Design review of the part shown in the three views and the two pictorial views. Dimensions are in mm from the part's minimum x, y and z. Coordinates: 2 decimals unless noted, no trailing zeros. Loops run counter-clockwise (first coordinate to the right, second up) from the corner with the lowest first, then second, coordinate; pieces in that order, holes last. Notation, with made-up numbers: (43, 51) -> (51, 51) arc R24 cw to (51, 72) -> close; hole circle Ø9 at (-37.75, -14). An arc over 180 degrees is marked (long way). Answer in a Markdown table with one row per item.
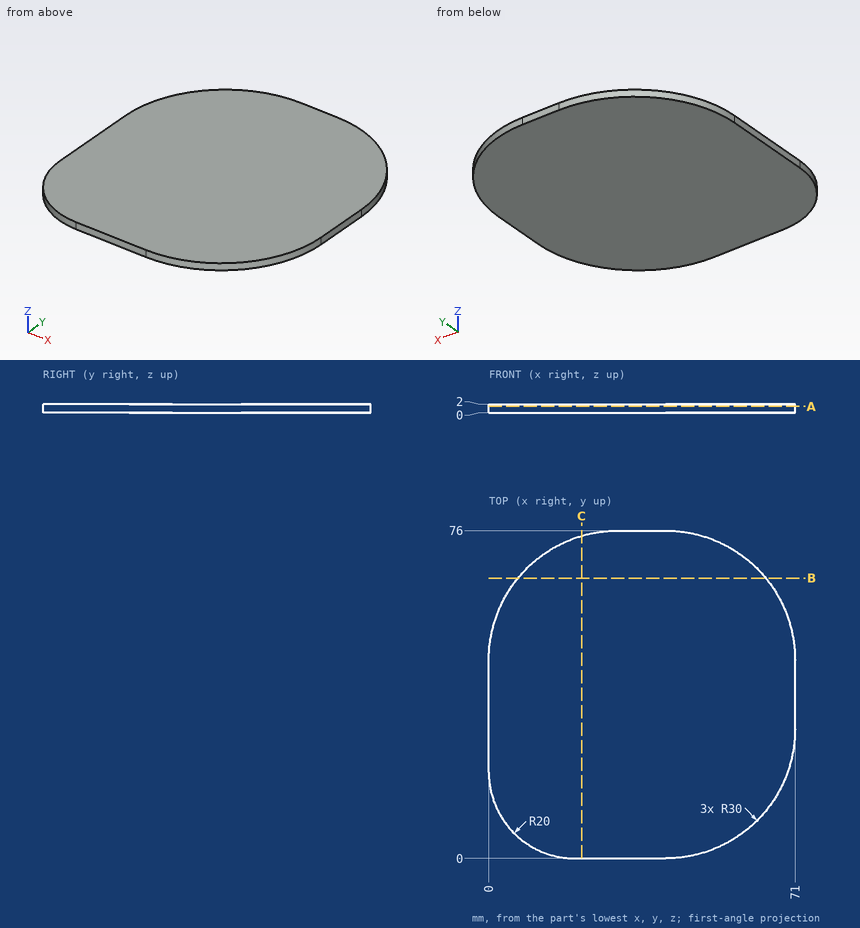
Item 1: For L1, parallel to X at y = 29.5, z = 0.1; L2, parallel to Y at x = 62, z = 1.2; L3, parallel to X at y = 71, z = 0.2, list the stretches that pass through material, from the lowest coordinate up.
Worked answers:
| item | result |
|---|---|
| L1 | 0 to 71 |
| L2 | 8.58 to 67.42 |
| L3 | 13.42 to 57.58 |
Item 2: Take a section at C-C, the plane x = 21.5. State the section outline as (y, z) points.
Worked answers:
| item | result |
|---|---|
| outline | (0, 0) -> (74.77, 0) -> (74.77, 2) -> (0, 2) -> close |
Item 3: Insertion check: pin 1 (1 mm diameter, centred on y = 12, z = 0.5, fed in from -X); pin 2 (1 mm diameter, centred on y = 56.5, z = 0.5, fed in from +X). Each pin has a flat end and moves straight along its axis. Give the tip position at first contact, or say it passes through.
Worked answers:
| item | result |
|---|---|
| pin 1 | x = 1.46 |
| pin 2 | x = 69.28 |
Item 4: Take a section at B-B, the plane y = 65. State the section outline as (x, z) points.
Worked answers:
| item | result |
|---|---|
| outline | (6.78, 0) -> (64.22, 0) -> (64.22, 2) -> (6.78, 2) -> close |
Item 5: Take a section at A-A, the plane z = 1.45. State the section outline as (x, y) points.
Worked answers:
| item | result |
|---|---|
| outline | (0, 20) arc R20 ccw to (20, 0) -> (41, 0) arc R30 ccw to (71, 30) -> (71, 46) arc R30 ccw to (41, 76) -> (30, 76) arc R30 ccw to (0, 46) -> close |
